Read the model definition and answer for the solid it produces. Units are mm, in the model's axes. A direction names the side the tool comes from. Give positions to 0.01 mm unless a question says otherwise; leave off trailing zeros. Order: outer loops, then holes, each group sorted by start corner. A loop starts at its lowest first (then second) coordinate and runs counter-clockwise, first axis right, second up. Notation, with made-up numbers: (72, 48) - (107, 48) arc R20 ccw to (107, 61) - close; hole circle Ø4 at (33.5, 69). An arc over 180 degrees is marked (long way). Use a Markdown table: item, result. Add a question column.
1. A cutting plane is placed at A-A on x = 0. Determine the outline of the cut face in (y, z), and give its area (3 significant figures).
2. A cutting plane is placed at C-C on y = 2.7. Determine the outline of the cut face in (x, z).
3. A cutting plane is placed at B-B on z = 0. Determine the outline of the cut face in (x, y) (1 decimal), and give its area (3 significant figures).
4. A cutting plane is placed at D-D on z = 3.75. Determine the outline of the cut face in (x, y), and give its area (3 significant figures).
5. Which of the six approach directions +Z, -Z, +X, -X, +Y, -Y give full straight-line access (tool end or side, diameter ignored) to faces 1 (the cylindrical face through (6.56, 0.64, 11.43)), 2 (the flat face through (7.337, 1, 0))?
6. Flat-ended cylindrical pins translate along their axes: P1, Ø0.5, axis at y = 1, z = -3, coming from the +X side; P2, Ø10.5, axis at x = -2.5, z = 1.5, coming from the -Y side; P3, Ø5, axis at x = -3, z = -7, coming from the +Y side. Find the tip coordinate at first contact, or state that the pin passes through.
7. For a pull along Z with two mould halves and no side action, classify faces 3 (the cylindrical face through (-1.294, 0.751, 5.827)), 4 (the cylindrical face through (-13.177, 0.64, -0.029)), 5 (the flat face through (-3.551, 0.751, -6.422)), 6 (the flat face through (-3.786, 0.751, 6.286)) as released by +Z, released by -Z, zero draft, split by the parting line, or undercut.
8. Consider L1, parallel to X at y = 0.6, z = 0; L2, parallel to Y at x = 0.75, z = -8; L3, parallel to X at y = 0.85, z = -4.5. Determine where each line is inside the solid, lowest interval first.
```python
from build123d import *

# Parameters (mm, degrees)
SKETCH1_R           = 5.969
BOSS_EXTRUDE1_DEPTH = 1.524
CIRPATTERN2_COUNT   = 3


with BuildPart() as part:
    # Sketch1 → Boss-Extrude1 (new body)
    with BuildSketch(Plane(origin=(0, 0, 0), x_dir=(1, 0, 0), z_dir=(0, 1, 0))):
        with BuildLine():
            Line((4.697427285, 11.184182722), (-12.0345, 1.524))
            ThreePointArc((-12.0345, 1.524), (-13.1775, 0), (-12.0345, -1.524))
            Line((-12.0345, -1.524), (4.697427285, -11.184182722))
            ThreePointArc((4.697427285, -11.184182722), (6.58875, -11.412049758), (7.337072715, -9.660182722))
            Line((7.337072715, -9.660182722), (7.337072715, 9.660182722))
            ThreePointArc((7.337072715, 9.660182722), (6.58875, 11.412049758), (4.697427285, 11.184182722))
        make_face()
        Circle(SKETCH1_R, mode=Mode.SUBTRACT)
    extrude(amount=BOSS_EXTRUDE1_DEPTH)

    # Sketch2 → Revolve1 (revolve)
    with BuildSketch(Plane(origin=(0, 1.524, 0), x_dir=(1, 0, 0), z_dir=(0, 1, 0))):
        with BuildLine():
            Line((-11.65220136, -1.5875), (-11.65220136, 1.5875))
            ThreePointArc((-11.65220136, 1.5875), (-10.06470136, 0), (-11.65220136, -1.5875))
        make_face()
    revolve1 = revolve(axis=Axis((-11.65220136, 1.524, 1.5875), (0, 0, -1)))

    # CirPattern2: Revolve1 ×3 about axis
    cirpattern2_axis = Axis((0, 0, 0), (0, 1, 0))
    for i in range(1, CIRPATTERN2_COUNT):
        add(revolve1.rotate(cirpattern2_axis, i * 360 / CIRPATTERN2_COUNT))


solid = part.part
```
Output values:
| question | item | result |
|---|---|---|
| 1 | outline | (0, -8.47) - (1.52, -8.47) - (1.52, -5.97) - (0, -5.97) - close; (0, 5.97) - (1.52, 5.97) - (1.52, 8.47) - (0, 8.47) - close |
| 1 | area | 7.63 mm² |
| 2 | outline | circle Ø2.13 at (-11.65, 0); circle Ø2.13 at (5.83, -10.09); circle Ø2.13 at (5.83, 10.09) |
| 3 | outline | (-13.2, 0) - (-12.1, 0) arc R1.6 ccw to (-11.2, 0) - (-6, 0) - (-6, 1.5) - (-10.1, 1.5) arc R1.6 ccw (long way) to (-13.2, 1.1) - close; (6, 0) - (7.3, 0) - (7.3, 1.5) - (6, 1.5) - close |
| 3 | area | 17.1 mm² |
| 4 | outline | (-8.18, 0) - (-4.64, 0) - (-4.64, 1.52) - (-8.18, 1.52) - close; (4.64, 0) - (7.34, 0) - (7.34, 1.52) - (4.64, 1.52) - close |
| 4 | area | 9.49 mm² |
| 5 | face 1 | -Y |
| 5 | face 2 | +X, +Y, -Y |
| 6 | P1 | x = 7.34 |
| 6 | P2 | y = 0 |
| 6 | P3 | y = 1.52 |
| 7 | face 3 | undercut |
| 7 | face 4 | split by the parting line |
| 7 | face 5 | released by -Z |
| 7 | face 6 | released by +Z |
| 8 | L1 | -13.18 to -5.97, 5.97 to 7.34 |
| 8 | L2 | 0 to 1.52 |
| 8 | L3 | -6.88 to -3.92, 3.92 to 7.34 |
